Could you check a few things on this model? Use its own coordinates, in mm. A direction names the side the tool comes from. Round coordinates to 2 decimals unless told otherwise and drop trailing zeros. Loops run counter-clockwise (first coordinate to the right, second up) from the corner with the lowest first, then second, coordinate; pieces in that order, holes last. Notation, with made-up numbers: M 15.25,-31.5 L 57.25,-31.5 A24 ccw 57.25,-10.5 Z; hole C -39.75,-35 d5. An arc over 180 degrees is marked long. Answer in a Markdown table with one row per item.
```python
from build123d import *

# Parameters (mm, degrees)
F0_R     = 12.7
F1_DEPTH = 25.4
F3_W     = 25.4
F3_H     = 381
F4_DEPTH = 25.4
F6_DEPTH = 50.8
F7_DEPTH = 25.4
F9_DEPTH = 25.4


with BuildPart() as f1:
    # F0 (on Top) → F1 (new body)
    with BuildSketch(Plane.XY):
        with Locations((-130.0663352013, -20.0254302472)):
            Circle(F0_R)
    extrude(amount=F1_DEPTH)


with BuildPart() as f4:
    # F3 (on Top) → F4 (new body)
    with BuildSketch(Plane.XY):
        with Locations((-44.869919461, 159.0675017536)):
            Rectangle(F3_W, F3_H)
    extrude(amount=F4_DEPTH)

    # F5 (on face) → F6 (join)
    with BuildSketch(Plane(origin=(0, 0, 0), x_dir=(1, 0, 0), z_dir=(0, 0, -1))):
        with BuildLine():
            ThreePointArc((-32.169919461, 6.0324982464), (-35.8896633399, 15.0127543675), (-44.869919461, 18.7324982464))
            ThreePointArc((-44.869919461, 18.7324982464), (-49.729999052, 17.7657683093), (-53.8501755821, 15.0127543675))
            Line((-53.8501755821, 15.0127543675), (-35.8896633399, -2.9477578746))
            ThreePointArc((-35.8896633399, -2.9477578746), (-33.1366493981, 1.1724186554), (-32.169919461, 6.0324982464))
        make_face()
        with BuildLine():
            ThreePointArc((-53.8501755821, 15.0127543675), (-56.6031895193, 10.8925778487), (-57.569919461, 6.0324982708))
            ThreePointArc((-57.569919461, 6.0324982708), (-53.8501755907, -2.947757866), (-44.869919461, -6.6675017536))
            ThreePointArc((-44.869919461, -6.6675017536), (-40.00983987, -5.7007718165), (-35.8896633399, -2.9477578746))
            Line((-35.8896633399, -2.9477578746), (-53.8501755821, 15.0127543675))
        make_face()
    extrude(amount=F6_DEPTH)

    # F7 (cut): a face of the model
    f7_faces = [f4.faces().sort_by_distance(p)[0] for p in [
        (-44.869919461, -6.0324982464, -50.8),
    ]]
    extrude(f7_faces, amount=-F7_DEPTH, mode=Mode.SUBTRACT)

    # F8 (on face) → F9 (join)
    with BuildSketch(Plane(origin=(0, 0, 0), x_dir=(1, 0, 0), z_dir=(0, 0, -1))):
        with BuildLine():
            ThreePointArc((-35.8896633399, -333.1477578746), (-33.1366493981, -329.0275813446), (-32.169919461, -324.1675017536))
            ThreePointArc((-32.169919461, -324.1675017536), (-35.8896633399, -315.1872456325), (-44.869919461, -311.4675017536))
            ThreePointArc((-44.869919461, -311.4675017536), (-49.729999052, -312.4342316907), (-53.8501755821, -315.1872456325))
            Line((-53.8501755821, -315.1872456325), (-35.8896633399, -333.1477578746))
        make_face()
        with BuildLine():
            ThreePointArc((-57.569919461, -324.1675017536), (-53.8501755821, -333.1477578746), (-44.869919461, -336.8675017536))
            ThreePointArc((-44.869919461, -336.8675017536), (-40.00983987, -335.9007718165), (-35.8896633399, -333.1477578746))
            Line((-35.8896633399, -333.1477578746), (-53.8501755821, -315.1872456325))
            ThreePointArc((-53.8501755821, -315.1872456325), (-56.6031895239, -319.3074221625), (-57.569919461, -324.1675017536))
        make_face()
    extrude(amount=F9_DEPTH)


solid = f4.part
```
1) Which directions (+Z, -Z, +X, -X, +Y, -Y) give clear straight access to the entire face, cutting with the end or side of a thin tool? Please do faces 1 (the face through (-45, 324, -25.4)), 2 (the face through (-45, -24, 0)).
Computed:
| item | result |
|---|---|
| face 1 | -Z, +X, -X, +Y, -Y |
| face 2 | -Z, -Y |
2) I want a section at C-C, the plane x = -39. Please give me the cut outline in (y, z), plus the area to 3 significant figures.
Computed:
| item | result |
|---|---|
| outline | M -31.43,0 L -17.29,0 L -17.29,-25.4 L 5.23,-25.4 L 5.23,0 L 312.91,0 L 312.91,-25.4 L 335.43,-25.4 L 335.43,0 L 349.57,0 L 349.57,25.4 L -31.43,25.4 Z |
| area | 10,800 mm² |
3) Will these pins go through, and if not, where does the flat tip stop? P1, Ø12, axis at x = -48, y = 112, coming from the -Z side; P2, Ø6, axis at x = -36, z = -5, coming from the -Y side; P3, Ø1.5, axis at x = -53.5, z = -10.5, coming from the -Y side.
Computed:
| item | result |
|---|---|
| P1 | stops at z = 0 |
| P2 | stops at y = -17.29 |
| P3 | stops at y = -15.99 |
4) If we mould it in two halves opening along Y, with no side actions, what happens to faces 3 (the face through (-45, 161, 0)), 4 (the face through (-45, 349.568, 13)), 5 (the face through (-57.57, 156, 13))? For each: released by +Y, released by -Y, zero draft, split by the parting line, or undercut.
Computed:
| item | result |
|---|---|
| face 3 | undercut |
| face 4 | released by +Y |
| face 5 | zero draft |
5) I want a section at A-A, the plane z = -10.5. Please give me the cut outline in (x, y).
Computed:
| item | result |
|---|---|
| outline | C -44.87,-6.03 d25.4; C -44.87,324.17 d25.4 |
6) I want a section at B-B, the plane y = 184. Please give me the cut outline in (x, z).
Computed:
| item | result |
|---|---|
| outline | M -57.57,0 L -32.17,0 L -32.17,25.4 L -57.57,25.4 Z |
7) I need wall thicknesses on line 1 (Y direction, x = -44, z = -18); line 2 (Z direction, x = -34, y = 239.5); line 3 (Y direction, x = -52.75, z = -1). Which ranges of each line are inside material? Lowest first, please.
Computed:
| item | result |
|---|---|
| line 1 | y = -18.7 to 6.64, 311.5 to 336.84 |
| line 2 | z = 0 to 25.4 |
| line 3 | y = -15.99 to 3.93, 314.21 to 334.13 |
